Here's how the part is built. I have some questions about the finished solid (model axes, mm). A direction names the side the tool comes from. Round coordinates to 2 decimals unless told otherwise and drop trailing zeros. Write each loop counter-clockwise with the first axis right and the second up, starting at its lowest first coordinate (ties: lowest second). Pieces come first, ordered by that corner, then holes. Notation, with made-up numbers: (-5, 36) - (15, 36) arc R28 ccw to (15, 67) - close; hole circle Ø1 at (53, 88.25). An arc over 180 degrees is marked (long way). Write item = value, one per line. Start each with the question number.
Item 1: For P1, Ø12, axis at x = -25, y = 10.5, coming from the -Z side; P2, Ø3.5, axis at x = -6, z = 6.5, coming from the +Y side; P3, Ø5, axis at x = 7.5, z = 7.5, coming from the -Y side; P4, Ø3.5, axis at y = 14.9, z = -2.85, coming from the -X side, each with a flat end and sliding along its axis, tell me the tip position at first contact or that it passes through.
Item 2: If I drill on line 1 along Z through (x, y) = (7.5, -0.25); line 2 along X through (y, z) = (27, 11.5); line 3 along Z through (x, y) = (-7.5, 1.2), over which ranges is the centre line in solid material (lowest first)? Write a range as [from, to].
Item 3: If we section it at B-B (z = 7.5): Please give me the cut outline in (x, y), and give its area (3 significant figures).
Item 4: If we section it at A-A (y = 23): Please give me the cut outline in (x, z), and give its area (3 significant figures).
Item 5: If we section it at D-D (z = 2.85): Give the number of separate pieces and of enclosed holes in the cut face, and give its area (3 significant figures).
Item 6: If we section it at C-C (x = -7.5): Please give me the cut outline in (y, z).
Item 7: Thinking about a two-plate mould opening in X: for faces 1 (the face through (-3.136, 0.961, 11.502)), 2 (the face through (31.074, 15.962, -3.29)), 3 (the face through (32.8, 16, 0)), which applies, pulls with the +X half, pulls with the -X half, needs draft (parallel to the pull), parting line crosses it, or undercut?
Item 8: Which directions (+Z, -Z, +X, -X, +Y, -Y) give clear straight access to the entire face, cutting with the end or side of a thin tool? Please do faces 4 (the face through (-10.445, -0.787, 8.427)), 5 (the face through (-28.8, 17, 7)), 6 (the face through (5, 0.15, -10)), 7 (the face through (-31, 17, 0)).
```python
from build123d import *

# Parameters (mm, degrees)
F0_W      = 65.6
F0_H      = 30
F1_DEPTH  = 1.75
F2_W      = 3.5
F2_H      = 31.5
F3_DEPTH  = 15
F4_W      = 4
F4_H      = 31
F5_DEPTH  = 15
F6_R      = 1.15
F7_DEPTH  = 200
F8_R      = 3.0875
F9_DEPTH  = 25
F10_R     = 5.9215
F11_DEPTH = 1.6


with BuildPart() as f1:
    # F0 (on Front) → F1 (new body, symmetric)
    with BuildSketch(Plane.XZ):
        Rectangle(F0_W, F0_H)
    extrude(amount=F1_DEPTH, both=True)

    # F2 (on Top) → F3 (join, symmetric)
    with BuildSketch(Plane.XY):
        with Locations((31.05, 17.5)):
            Rectangle(F2_W, F2_H)
    extrude(amount=F3_DEPTH, both=True)

    # F4 (on Top) → F5 (join)
    with BuildSketch(Plane.XY):
        with Locations((-30.8, 17.25)):
            Rectangle(F4_W, F4_H)
    extrude(amount=F5_DEPTH)

    # F6 (on face) → F7 (cut)
    with BuildSketch(Plane.YZ.offset(32.8)):
        with Locations((14.9, 2.85)):
            Circle(F6_R)
        with Locations((20.6, 2.85)):
            Circle(F6_R)
        with Locations((14.9, -2.85)):
            Circle(F6_R)
        with Locations((20.6, -2.85)):
            Circle(F6_R)
    extrude(amount=-F7_DEPTH, mode=Mode.SUBTRACT)

    # F8 (on face) → F9 (cut)
    with BuildSketch(Plane(origin=(0, 1.75, 0), x_dir=(-1, 0, 0), z_dir=(0, 1, 0))):
        with Locations((-7.5, 7.5)):
            Circle(F8_R)
        with Locations((-7.5, -7.5)):
            Circle(F8_R)
        with Locations((7.5, 7.5)):
            Circle(F8_R)
        with Locations((7.5, -7.5)):
            Circle(F8_R)
    extrude(amount=-F9_DEPTH, mode=Mode.SUBTRACT)

    # F10 (on face) → F11 (cut)
    with BuildSketch(Plane(origin=(0, 1.75, 0), x_dir=(-1, 0, 0), z_dir=(0, 1, 0))):
        with Locations((-7.5, 7.5)):
            Circle(F10_R)
        with Locations((-7.5, -7.5)):
            Circle(F10_R)
        with Locations((7.5, -7.5)):
            Circle(F10_R)
        with Locations((7.5, 7.5)):
            Circle(F10_R)
    extrude(amount=-F11_DEPTH, mode=Mode.SUBTRACT)


solid = f1.part
```
Reply:
q1.P1 = 0
q1.P2 = 0.15
q1.P3 = through
q1.P4 = 29.3
q2.line_1 = [-15, -10.59], [-4.41, 4.41], [10.59, 15]
q2.line_2 = [-32.8, -28.8], [29.3, 32.8]
q2.line_3 = [-15, -13.42], [-1.58, 1.58], [13.42, 15]
q3.outline = (-32.8, -1.75) - (-10.59, -1.75) - (-10.59, 0.15) - (-13.42, 0.15) - (-13.42, 1.75) - (-28.8, 1.75) - (-28.8, 32.75) - (-32.8, 32.75) - close; (-4.41, -1.75) - (4.41, -1.75) - (4.41, 0.15) - (1.58, 0.15) - (1.58, 1.75) - (-1.58, 1.75) - (-1.58, 0.15) - (-4.41, 0.15) - close; (10.59, -1.75) - (32.8, -1.75) - (32.8, 33.25) - (29.3, 33.25) - (29.3, 1.75) - (13.42, 1.75) - (13.42, 0.15) - (10.59, 0.15) - close
q3.area = 402 mm2
q4.outline = (-32.8, 0) - (-28.8, 0) - (-28.8, 15) - (-32.8, 15) - close; (29.3, -15) - (32.8, -15) - (32.8, 15) - (29.3, 15) - close
q4.area = 165 mm2
q5.separate_pieces = 5
q5.enclosed_holes = 0
q5.area = 406 mm2
q6.outline = (-1.75, -15) - (1.75, -15) - (1.75, -13.42) - (0.15, -13.42) - (0.15, -10.59) - (-1.75, -10.59) - close; (-1.75, -4.41) - (0.15, -4.41) - (0.15, -1.58) - (1.75, -1.58) - (1.75, 1.58) - (0.15, 1.58) - (0.15, 4.41) - (-1.75, 4.41) - close; (-1.75, 10.59) - (0.15, 10.59) - (0.15, 13.42) - (1.75, 13.42) - (1.75, 15) - (-1.75, 15) - close
q7.face_1 = undercut
q7.face_2 = needs draft
q7.face_3 = pulls with the +X half
q8.face_4 = +Y, -Y
q8.face_5 = +Z, -Z, +Y
q8.face_6 = +Y
q8.face_7 = -Z, -X, +Y
